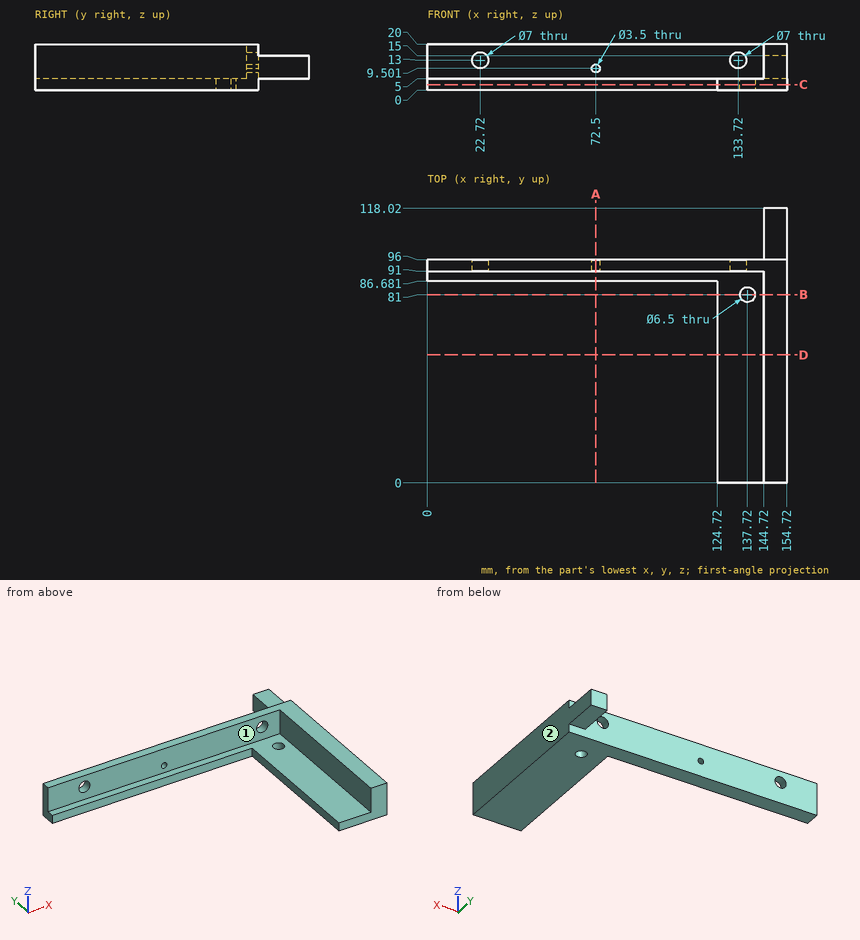
Could you check a few things on this drawing? It's one solid part, dimensions in mm from its lowest x, y, z. A direction names the side the tool comes from. Round coordinates to 2 decimals unless told otherwise and drop trailing zeros. Order: outer loops, then holes, each group sorted by start corner. A loop starts at its lowest first (then second) coordinate and runs counter-clockwise, first axis right, second up. Notation, with made-up numbers: M 38,88 L 67,88 A26 cw 67,109 Z; hole C 18.5,-27 d11. An arc over 180 degrees is marked long. One line per item, written item: value.
(1) Imagine slicing it at C-C (z = 2.5). Write out the boundary of the cut face in (x, y).
Ans:
outline: M 0,86.68 L 124.72,86.68 L 124.72,0 L 154.72,0 L 154.72,96 L 0,96 Z; hole C 137.72,81 d6.5
(2) Imagine slicing it at D-D (y = 55). Write out the boundary of the cut face in (x, z), and give its area (3 significant figures).
Ans:
outline: M 124.72,0 L 154.72,0 L 154.72,20 L 144.72,20 L 144.72,5 L 124.72,5 Z
area: 300 mm^2
(3) Imagine slicing it at A-A (x = 72.5). Write out the boundary of the cut face in (y, z).
Ans:
outline: M 86.68,0 L 96,0 L 96,7.75 L 91,7.75 L 91,5 L 86.68,5 Z; M 91,11.25 L 96,11.25 L 96,20 L 91,20 Z
(4) I need wall thicknesses on line 1 along X through (y, z) = (93.35, 13); line 2 along X through (y, z) = (22, 4.25); line 3 along Z through (x, y) = (37.5, 90.5). Which ranges of each line are inside material? Lowest first, please. Write a range as from..to.
Ans:
line 1: x = 0..19.22, 26.22..130.22, 137.22..154.72
line 2: x = 124.72..154.72
line 3: z = 0..5
(5) Which directions (+Z, -Z, +X, -X, +Y, -Y) give clear straight access to the entire face, cutting with the end or side of a thin tool? Please do the marked faces 1 and 2.
Ans:
face 1: +Z, -X, -Y
face 2: +Z, -Z, +X, +Y, -Y
(6) Imagine slicing it at B-B (y = 81). Write out the boundary of the cut face in (x, z).
Ans:
outline: M 124.72,0 L 134.47,0 L 134.47,5 L 124.72,5 Z; M 140.97,0 L 154.72,0 L 154.72,20 L 144.72,20 L 144.72,5 L 140.97,5 Z
(7) I'm going to push flat-ended pins straight in: P1, Ø5, axis at y = 55, z = 12, coming from the -X side; P2, Ø3, axis at x = 149.5, y = 109, coming from the +Z side; P3, Ø8, axis at y = 99, z = 4.5, coming from the +X side; P4, Ø8, axis at x = 22.72, z = 13, coming from the +Y side. Where does each tip first touch, or does it pass through?
Ans:
P1: stops at x = 144.72
P2: stops at z = 15
P3: stops at x = 154.72
P4: stops at y = 96
